Autodesk Inventor part; units mm, degrees
ref_plane "YZ Plane" through (0, 0, 0) normal (1, 0, 0) x (0, 1, 0)
ref_plane "XZ Plane" through (0, 0, 0) normal (0, 1, 0) x (-1, 0, 0)
ref_plane "XY Plane" through (0, 0, 0) normal (0, 0, 1) x (1, 0, 0)
sketch "草圖1" plane through (0, 0, 0) normal (0, 0, 1) x (1, 0, 0)
  line L0 (-23.85, -77.5) -> (23.85, 77.5) construction
  line L1 (23.85, -77.5) -> (-23.85, 77.5) construction
  line L2 (0, 127.6921) -> (0, -161.3915) construction
  line L3 (-23.85, 75.5) -> (-23.85, -75.5)
  line L4 (23.85, -75.5) -> (23.85, 75.5)
  line L5 (-5, 24.5) -> (5, 24.5)
  line L6 (7, 26.5) -> (7, 75.5)
  line L7 (-7, 75.5) -> (-7, 26.5)
  line L8 (-7, 24.5) -> (7, 77.5) construction
  line L9 (7, 24.5) -> (-7, 77.5) construction
  line L10 (21.85, 77.5) -> (9, 77.5)
  line L11 (-9, 77.5) -> (-21.85, 77.5)
  arc A0 (-7, 75.5) -> (-9, 77.5) centre (-9, 75.5) ccw
  arc A1 (9, 77.5) -> (7, 75.5) centre (9, 75.5) ccw
  arc A2 (-7, 26.5) -> (-5, 24.5) centre (-5, 26.5) ccw
  arc A3 (5, 24.5) -> (7, 26.5) centre (5, 26.5) ccw
  arc A4 (-21.85, 77.5) -> (-23.85, 75.5) centre (-21.85, 75.5) ccw
  arc A5 (23.85, 75.5) -> (21.85, 77.5) centre (21.85, 75.5) ccw
  line L12 (-82.8249, 0) -> (86.4934, 0) construction
  line L13 (-5, -24.5) -> (5, -24.5)
  line L14 (7, -26.5) -> (7, -75.5)
  line L15 (-7, -75.5) -> (-7, -26.5)
  line L16 (-7, -24.5) -> (7, -77.5) construction
  line L17 (7, -24.5) -> (-7, -77.5) construction
  line L18 (21.85, -77.5) -> (9, -77.5)
  line L19 (-9, -77.5) -> (-21.85, -77.5)
  arc A6 (-9, -77.5) -> (-7, -75.5) centre (-9, -75.5) ccw
  arc A7 (7, -75.5) -> (9, -77.5) centre (9, -75.5) ccw
  arc A8 (-5, -24.5) -> (-7, -26.5) centre (-5, -26.5) ccw
  arc A9 (7, -26.5) -> (5, -24.5) centre (5, -26.5) ccw
  arc A10 (-23.85, -75.5) -> (-21.85, -77.5) centre (-21.85, -75.5) ccw
  arc A11 (21.85, -77.5) -> (23.85, -75.5) centre (21.85, -75.5) ccw
  line L20 (-21.85, -77.5) -> (-9, -77.5)
  line L21 (9, -77.5) -> (21.85, -77.5)
  line L22 (-6.85, -17.45) -> (6.85, -17.45)
  line L23 (6.85, 16.75) -> (-6.85, 16.75)
  line L24 (12.065, 0.7) -> (12.065, 6.7)
  line L25 (-12.065, 6.7) -> (-12.065, 0.7)
  line L26 (-12.065, 0.7) -> (12.065, 6.7) construction
  line L27 (12.065, 0.7) -> (-12.065, 6.7) construction
  line L28 (-6.85, 16.75) -> (-6.85, 6.7)
  line L29 (6.85, 6.7) -> (6.85, 16.75)
  line L30 (12.065, 6.7) -> (6.85, 6.7)
  line L31 (7.85, 0.7) -> (12.065, 0.7)
  line L32 (-12.065, 0.7) -> (-7.85, 0.7)
  line L33 (-6.85, 6.7) -> (-12.065, 6.7)
  line L34 (-7.85, 0.7) -> (-7.85, -5.3)
  line L35 (-7.85, -5.3) -> (-6.85, -5.3)
  line L36 (-6.85, -5.3) -> (-6.85, -17.45)
  line L37 (7.85, 0.7) -> (7.85, -5.3)
  line L38 (7.85, -5.3) -> (6.85, -5.3)
  line L39 (6.85, -17.45) -> (6.85, -5.3)
  point P0 (0, 0)
  point P1 (0, 51)
  point P2 (0, -51)
  point P3 (0, 3.7)
  point P4 (12.065, 3.7)
  point P5 (-23.85, -75.5)
  dimension "d0" = 47.7
  dimension "d22" = 14
  dimension "d24" = 2
  dimension "d25" = 2
  dimension "d26" = 34.2
  dimension "d27" = 13.7
  dimension "d28" = 6
  dimension "d30" = 24.13
  dimension "d31" = 10.05
  dimension "d54" = 53
  dimension "d97" = 6
  dimension "d98" = 1
  dimension "d101" = 0.7
  dimension "d103" = 155
extrude "擠出1" add sketch "草圖1" along normal blind 3
sketch "草圖3" plane through (0, 0, 3) normal (0, 0, 1) x (1, 0, 0)
  line L0 (-88.1264, 0) -> (75.7938, 0)
  line L1 (0, 123.8394) -> (0, -129.4918)
  point P0 (0, 0)
sketch "草圖5" plane through (0, 0, 3) normal (0, 0, 1) x (1, 0, 0)
  line L0 (-9.85, -17.45) -> (-13.85, -17.45)
  line L1 (-13.85, -17.45) -> (-13.85, -14.45)
  line L2 (-13.85, -14.45) -> (-9.85, -14.45)
  line L3 (-9.85, -14.45) -> (-9.85, -17.45)
  line L4 (6.85, -17.45) -> (-6.85, -17.45)
  line L5 (-9.85, 13.75) -> (-13.85, 13.75)
  line L6 (-13.85, 13.75) -> (-13.85, 16.75)
  line L7 (-13.85, 16.75) -> (-9.85, 16.75)
  line L8 (-9.85, 16.75) -> (-9.85, 13.75)
  line L9 (-6.85, 16.75) -> (6.85, 16.75)
  line L10 (0, 31.1544) -> (0, -25.4134)
  line L11 (9.85, -17.45) -> (13.85, -17.45)
  line L12 (13.85, -17.45) -> (13.85, -14.45)
  line L13 (13.85, -14.45) -> (9.85, -14.45)
  line L14 (9.85, -14.45) -> (9.85, -17.45)
  line L15 (13.85, 16.75) -> (9.85, 16.75)
  line L16 (13.85, 13.75) -> (13.85, 16.75)
  line L17 (9.85, 13.75) -> (13.85, 13.75)
  line L18 (9.85, 16.75) -> (9.85, 13.75)
  line L19 (-17.85, 1.825) -> (-20.85, 1.825)
  line L20 (-20.85, 1.825) -> (-20.85, 13.825)
  line L21 (-20.85, 13.825) -> (-17.85, 13.825)
  line L22 (-17.85, 13.825) -> (-17.85, 1.825)
  line L23 (17.85, 1.825) -> (20.85, 1.825)
  line L24 (20.85, 1.825) -> (20.85, 13.825)
  line L25 (20.85, 13.825) -> (17.85, 13.825)
  line L26 (17.85, 13.825) -> (17.85, 1.825)
  line L27 (-6.85, -17.45) -> (-6.85, 16.75) construction
  point P0 (0, 0)
  dimension "d60" = 4
  dimension "d62" = 3
  dimension "d64" = 3
  dimension "d66" = 3
  dimension "d67" = 12
  dimension "d96" = 3
  dimension "d100" = 11
  dimension "d102" = 0.075
extrude "擠出4" cut sketch "草圖5" against normal up to next
properties part number "main_frame" material "木材 (楓木)"
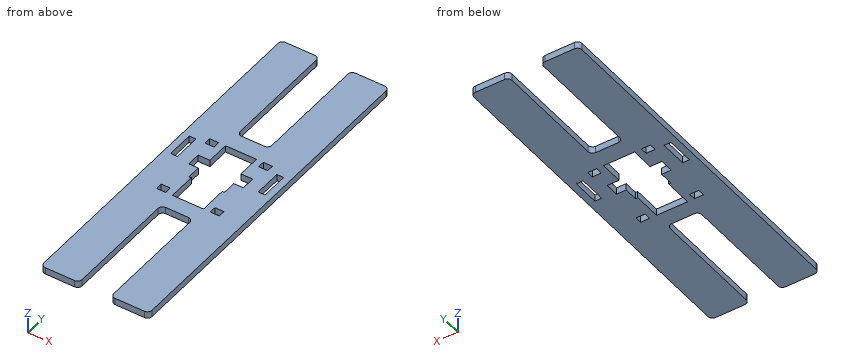
Geometry check sheet. Reference: the model listing, model coordinates, mm. Coordinates: 2 decimals unless noted, no trailing zeros. Loops run counter-clockwise (first coordinate to the right, second up) from the corner with the lowest first, then second, coordinate; pieces in that order, holes last. Notation, with made-up numbers: (41, 80.25) -> (61, 80.25) arc R20 cw to (61, 90.25) -> close; hole circle Ø3 at (16, 64.5). An arc over 180 degrees is marked (long way). Put each result on its own line as item: value.
1) Cross-section at C-C on y = 59.5. Record the boundary of the cut face in (x, z), plus the area to 3 significant figures.
Result set:
outline: (-23.85, 0) -> (-7, 0) -> (-7, 3) -> (-23.85, 3) -> close; (7, 0) -> (23.85, 0) -> (23.85, 3) -> (7, 3) -> close
area: 101 mm^2
2) Thickness scan on line 1 (Y direction, x = 20.5, z = 1.7) (3 decimals); line 2 (Y direction, x = 3, z = 1.95); line 3 (X direction, y = -30, z = 0.9). Record the ranges inside material, lowest first.
Result set:
line 1: y = -77.5 to 1.825, 13.825 to 77.5
line 2: y = -24.5 to -17.45, 16.75 to 24.5
line 3: x = -23.85 to -7, 7 to 23.85
3) Gauge pin test, flat ends, axial feed: pin 1 Ø8 at (x, y) = (6.5, 52) entering from +Z; pin 2 Ø1.1 at (x, z) = (-7.5, 2) entering from +Y; pin 3 Ø0.9 at (x, z) = (2, 2) entering from -Y. Record the tip position at first contact, or that the pin passes through.
Result set:
pin 1: stops at z = 3
pin 2: stops at y = 77.26
pin 3: stops at y = -24.5
4) Cross-section at D-D on z = 1.05. Count the separate pieces of the cut face and the enclosed holes in it, plus the area to 3 significant figures.
Result set:
separate pieces: 1
enclosed holes: 7
area: 5,240 mm^2
5) Cross-section at A-A on y = 4. Record the boundary of the cut face in (x, z) (3 decimals).
Result set:
outline: (-23.85, 0) -> (-20.85, 0) -> (-20.85, 3) -> (-23.85, 3) -> close; (-17.85, 0) -> (-12.065, 0) -> (-12.065, 3) -> (-17.85, 3) -> close; (12.065, 0) -> (17.85, 0) -> (17.85, 3) -> (12.065, 3) -> close; (20.85, 0) -> (23.85, 0) -> (23.85, 3) -> (20.85, 3) -> close
6) Cross-section at B-B on x = -1. Record the boundary of the cut face in (y, z), plus the area to 3 significant figures.
Result set:
outline: (-24.5, 0) -> (-17.45, 0) -> (-17.45, 3) -> (-24.5, 3) -> close; (16.75, 0) -> (24.5, 0) -> (24.5, 3) -> (16.75, 3) -> close
area: 44.4 mm^2
